Here's how the part is built. I have some questions about the finished solid (model axes, mm). Face numbers are marked on the shaded views. Round coordinates to 2 decimals unless told otherwise and drop trailing zeros. Write each loop counter-clockwise with the first axis right and the second up, starting at its lowest first coordinate (ties: lowest second). Pieces come first, ordered by that corner, then holes. Notation, with made-up numbers: M 26,-25 L 68,-25 A15 ccw 68,-15 Z; hole C 30,72 d11. An arc over 180 degrees is marked long. Use a Markdown table: item, result. Add a question column.
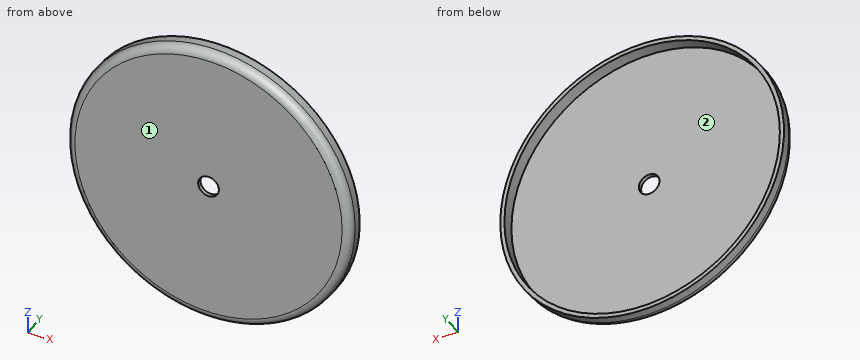
```python
from build123d import *

# Parameters (mm, degrees)
SKETCH1_R           = 42.291
SKETCH1_R_2         = 3.175
BOSS_EXTRUDE1_DEPTH = 1.27
SKETCH2_R           = 43.561
SKETCH2_R_2         = 42.291
BOSS_EXTRUDE2_DEPTH = 5.08
FILLET1_R           = 2.54


with BuildPart() as part:
    # Sketch1 → Boss-Extrude1 (new body)
    with BuildSketch(Plane(origin=(0, 0, 0), x_dir=(1, 0, 0), z_dir=(0, 1, 0))):
        Circle(SKETCH1_R)
        Circle(SKETCH1_R_2, mode=Mode.SUBTRACT)
    extrude(amount=BOSS_EXTRUDE1_DEPTH)

    # Sketch2 → Boss-Extrude2 (add)
    with BuildSketch(Plane.XZ):
        Circle(SKETCH2_R)
        Circle(SKETCH2_R_2, mode=Mode.SUBTRACT)
    extrude(amount=-BOSS_EXTRUDE2_DEPTH)

    # Fillet1
    fillet1_edges = [part.edges().sort_by_distance(p)[0] for p in [
        (-43.561, 0, 0),
    ]]
    fillet(fillet1_edges, radius=FILLET1_R)


solid = part.part
```
Item 1: I need wall thicknesses on probe 1 along Z at (x, y) = (0, 3.25); probe 2 along Z at (x, y) = (0, 2.3); probe 3 along Y at (x, z) = (-34.5, 5.5). Which ranges of each line are inside material? Lowest first, please. Write a range as from..to.
Item 2: Imagine slicing it at A-A on z = 0. List the corners of the cut face in (x, y) for me (3 decimals).
Item 3: Imagine slicing it at B-B on x = 0. List the corners of the cut face in (y, z) for me (3 decimals), plus the area to 3 significant figures.
Item 4: If we mould it in two halves opening along Z, with no side actions, what happens to the marked faces 1 and 2? For each: +Z half, -Z half, draft (parallel to the pull), parting line (faces both ways), or undercut.
Item 5: For pin 1 Ø2 at (x, y) = (-2.5, 2.5) entering from -Z; pin 2 Ø4 at (x, z) = (0, 0) entering from +Y, each with a flat end and sliding along its axis, tell me the tip position at first contact or that it passes through.
Item 6: Imagine slicing it at C-C on y = 4. List the corners of the cut face in (x, z) for me, plus the area to 3 significant figures.
The answers:
| question | item | result |
|---|---|---|
| 1 | probe 1 | -43.56..-42.29, 42.29..43.56 |
| 1 | probe 2 | -43.55..-42.29, 42.29..43.55 |
| 1 | probe 3 | 0..1.27 |
| 2 | outline | M -43.561,2.54 A2.54 ccw -41.021,0 L -3.175,0 L -3.175,1.27 L -42.291,1.27 L -42.291,5.08 L -43.561,5.08 Z; M 3.175,0 L 41.021,0 A2.54 ccw 43.561,2.54 L 43.561,5.08 L 42.291,5.08 L 42.291,1.27 L 3.175,1.27 Z |
| 3 | outline | M 0,-41.021 A2.54 ccw 2.54,-43.561 L 5.08,-43.561 L 5.08,-42.291 L 1.27,-42.291 L 1.27,-3.175 L 0,-3.175 Z; M 0,3.175 L 1.27,3.175 L 1.27,42.291 L 5.08,42.291 L 5.08,43.561 L 2.54,43.561 A2.54 ccw 0,41.021 Z |
| 3 | area | 109 mm² |
| 4 | face 1 | draft |
| 4 | face 2 | undercut |
| 5 | pin 1 | z = -43.54 |
| 5 | pin 2 | through |
| 6 | outline | C 0,0 d87.12; hole C 0,0 d84.58 |
| 6 | area | 343 mm² |
